For this review, take the finished solid that the model builds, in its own axes (mm). Face numbers are marked on the shaded views. A direction names the side the tool comes from. Coordinates: 2 decimals unless noted, no trailing zeros. Order: outer loops, then holes, each group sorted by start corner. A loop starts at its lowest first (then second) coordinate and runs counter-clockwise, first axis right, second up. Notation, with made-up numbers: (21.25, 12) -> (39.25, 12) arc R19 ccw to (39.25, 31) -> close; hole circle Ø3 at (81, -38). An arc over 180 degrees is marked (long way). Answer as a JSON object with one key per item and string values. Group by question number.
1) Draft analysis for pull direction X (two halves, no side actions). For the marked faces 5, 6, 7 and 8, state which applies: +X half, -X half, draft (parallel to the pull), parting line (faces both ways), or undercut.
2) Machinability: for the marked faces 1, 2, 3 and 4, which of the approach directions +Z, -Z, +X, -X, +Y, -Y give a long, thin tool a straight path to every point of the face, cutting with its end or side? Answer none if there is none.
3) Add section D-D, the plane z = 17.5. Write out the cut boundary in (x, y).
4) For pin 1 (1.5 mm diameter, centred on x = 9.5, z = 26.5, fed in from +Y); pin 2 (2 mm diameter, centred on x = -30, y = -15, fed in from -Z), all flat-tipped, find the tip position at first contact; note any pin that passes through.
5) Add section B-B, the plane z = 31. Write out the cut boundary in (x, y), then the cut area to 3 significant figures.
6) Wall thickness on L1, parallel to Y at x = 20, z = 18; L2, parallel to Y at x = -42.5, z = 5; L3, parallel to X at y = -7, z = 31: over which ranges is each line inside the solid? List them lowest first.
7) Add section A-A, the plane x = 1. Write out the cut boundary in (y, z).
8) Add section C-C, the plane y = 10. Write out the cut boundary in (x, z), then the cut area to 3 significant figures.
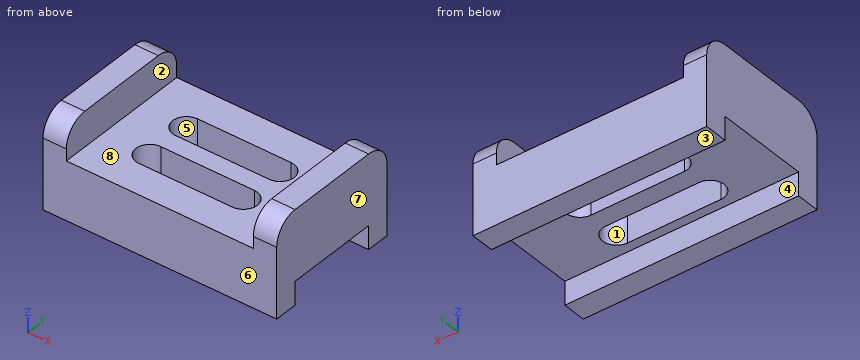
from build123d import *

# Parameters (mm, degrees)
F0_W     = 100
F0_H     = 60
F1_DEPTH = 40
F2_W     = 40
F2_H     = 10
F3_DEPTH = 100.001
F4_W     = 80
F4_H     = 60
F5_DEPTH = 15
F7_DEPTH = 25.001
F8_R     = 10


with BuildPart() as f1:
    # F0 (on Top) → F1 (new body)
    with BuildSketch(Plane.XY):
        Rectangle(F0_W, F0_H)
    extrude(amount=F1_DEPTH)

    # F2 (on face) → F3 (cut, through all)
    with BuildSketch(Plane.YZ.offset(50)):
        with Locations((0, 5)):
            Rectangle(F2_W, F2_H)
    extrude(amount=-F3_DEPTH, mode=Mode.SUBTRACT)

    # F4 (on face) → F5 (cut)
    with BuildSketch(Plane.XY.offset(40)):
        Rectangle(F4_W, F4_H)
    extrude(amount=-F5_DEPTH, mode=Mode.SUBTRACT)

    # F6 (on face) → F7 (cut, through all)
    with BuildSketch(Plane.XY.offset(25)):
        with BuildLine():
            Line((20, 16), (-20, 16))
            ThreePointArc((-20, 16), (-26, 10), (-20, 4))
            Line((-20, 4), (20, 4))
            ThreePointArc((20, 4), (26, 10), (20, 16))
        make_face()
        with BuildLine():
            Line((20, -4), (-20, -4))
            ThreePointArc((-20, -4), (-26, -10), (-20, -16))
            Line((-20, -16), (20, -16))
            ThreePointArc((20, -16), (26, -10), (20, -4))
        make_face()
    extrude(amount=-F7_DEPTH, mode=Mode.SUBTRACT)

    # F8
    f8_edges = [f1.edges().sort_by_distance(p)[0] for p in [
        (45, -30, 40),
        (-45, -30, 40),
        (45, 30, 40),
        (-45, 30, 40),
    ]]
    fillet(f8_edges, radius=F8_R)


solid = f1.part
Output values:
{
 "1": {"face 5": "undercut", "face 6": "draft", "face 7": "+X half", "face 8": "undercut"},
 "2": {"face 1": "+Z, -Z", "face 2": "+Z, +Y, -Y", "face 3": "-Z, +X, -X, +Y, -Y", "face 4": "-Z, +X, -X"},
 "3": {"outline": "(-50, -30) -> (50, -30) -> (50, 30) -> (-50, 30) -> close; hole (-20, -16) -> (20, -16) arc R6 ccw to (20, -4) -> (-20, -4) arc R6 ccw to start; hole (-20, 4) -> (20, 4) arc R6 ccw to (20, 16) -> (-20, 16) arc R6 ccw to start"},
 "4": {"pin 1": "passes through", "pin 2": "stops at z = 10"},
 "5": {"outline": "(-50, -29.95) -> (-40, -29.95) -> (-40, 29.95) -> (-50, 29.95) -> close; (40, -29.95) -> (50, -29.95) -> (50, 29.95) -> (40, 29.95) -> close", "area": "1,200 mm²"},
 "6": {"L1": "y = -30 to -16, -4 to 4, 16 to 30", "L2": "y = -30 to -20, 20 to 30", "L3": "x = -50 to -40, 40 to 50"},
 "7": {"outline": "(-30, 0) -> (-20, 0) -> (-20, 10) -> (-16, 10) -> (-16, 25) -> (-30, 25) -> close; (-4, 10) -> (4, 10) -> (4, 25) -> (-4, 25) -> close; (16, 10) -> (20, 10) -> (20, 0) -> (30, 0) -> (30, 25) -> (16, 25) -> close"},
 "8": {"outline": "(-50, 10) -> (-26, 10) -> (-26, 25) -> (-40, 25) -> (-40, 40) -> (-50, 40) -> close; (26, 10) -> (50, 10) -> (50, 40) -> (40, 40) -> (40, 25) -> (26, 25) -> close", "area": "1,020 mm²"}
}
